Here's how the part is built. I have some questions about the finished solid (model axes, mm). Face numbers are marked on the shaded views. A direction names the side the tool comes from. Coordinates: 2 decimals unless noted, no trailing zeros. Write each loop counter-clockwise with the first axis right and the second up, starting at its lowest first coordinate (ties: lowest second). Pieces come first, ordered by that corner, then holes.
```python
from build123d import *

# Parameters (mm, degrees)
SKETCH1_R           = 2.413
BOSS_EXTRUDE1_DEPTH = 6.35


with BuildPart() as part:
    # Sketch1 → Boss-Extrude1 (new body)
    with BuildSketch(Plane(origin=(0, 0, 0), x_dir=(1, 0, 0), z_dir=(0, 1, 0))):
        Polygon((-44.45, -12.7), (-31.75, -12.7), (-25.4, -12.7), (-25.4, -19.05), (-12.7, -19.05), (-12.7, -12.7), (0, -12.7), (0, -19.05), (12.7, -19.05), (12.7, -12.7), (31.75, -12.7), (31.75, 12.7), (12.7, 12.7), (12.7, 19.05), (0, 19.05), (0, 12.7), (-12.7, 12.7), (-12.7, 19.05), (-25.4, 19.05), (-25.4, 12.7), (-31.75, 12.7), (-44.45, 12.7), align=None)
        with Locations((-6.35, 0)):
            Circle(SKETCH1_R, mode=Mode.SUBTRACT)
    extrude(amount=BOSS_EXTRUDE1_DEPTH)


solid = part.part
```
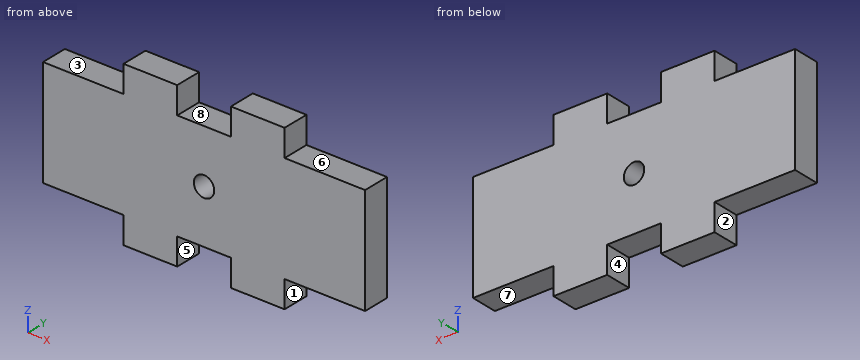
1) On a 3-axis mill with a long thin cutter (end or side, diameter ignored), from which of +Z, -Z, +X, -X, +Y, -Y can I reach the whole of each face in a straight line? I mean the marked faces 5, 6, 7 and 8. Say none if no direction works.
Values follow:
face 5: -Z, +Y, -Y
face 6: +Z, +X, +Y, -Y
face 7: -Z, +X, +Y, -Y
face 8: +Z, +Y, -Y
2) We'd pull the mould along X, two halves only. Please class the marked faces 1, 2, 3 and 4: pulls with the +X half, pulls with the -X half, needs draft (parallel to the pull), parting line crosses it, or undercut.
Values follow:
face 1: pulls with the +X half
face 2: pulls with the -X half
face 3: needs draft
face 4: undercut
3) I need wall thicknesses on probe 1 along X at (y, z) = (2.75, 13); probe 2 along Z at (x, y) = (-6.35, 1.5); probe 3 along X at (y, z) = (2, 0). Which ranges of each line are inside material? Lowest first, please.
Values follow:
probe 1: x = -25.4 to -12.7, 0 to 12.7
probe 2: z = -12.7 to -2.41, 2.41 to 12.7
probe 3: x = -44.45 to -8.76, -3.94 to 31.75
4) Imagine slicing it at B-B on z = 16. Please give me the cut outline in (x, y).
Values follow:
outline: (-25.4, 0) - (-12.7, 0) - (-12.7, 6.35) - (-25.4, 6.35) - close; (0, 0) - (12.7, 0) - (12.7, 6.35) - (0, 6.35) - close
5) Will these pins go through, and if not, where does the flat tip stop? pin 1 (5 mm diameter, centred on x = -32, z = 11.5, fed in from -Y); pin 2 (1.5 mm diameter, centred on x = 13.5, y = 2, fed in from -Z); pin 3 (3 mm diameter, centred on y = 3.5, z = 16.5, fed in from +X); pin 4 (1.9 mm diameter, centred on x = -36, y = 2, fed in from +Z).
Values follow:
pin 1: stops at y = 0
pin 2: stops at z = -12.7
pin 3: stops at x = 12.7
pin 4: stops at z = 12.7
6) Imagine slicing it at A-A on x = -6.35. Please give me the cut outline in (y, z), then the cut area to 3 significant figures.
Values follow:
outline: (0, -12.7) - (6.35, -12.7) - (6.35, -2.41) - (0, -2.41) - close; (0, 2.41) - (6.35, 2.41) - (6.35, 12.7) - (0, 12.7) - close
area: 131 mm2
7) Imagine slicing it at C-C on y = 2.25. Please give me the cut outline in (x, z), then the cut area to 3 significant figures.
Values follow:
outline: (-44.45, -12.7) - (-25.4, -12.7) - (-25.4, -19.05) - (-12.7, -19.05) - (-12.7, -12.7) - (0, -12.7) - (0, -19.05) - (12.7, -19.05) - (12.7, -12.7) - (31.75, -12.7) - (31.75, 12.7) - (12.7, 12.7) - (12.7, 19.05) - (0, 19.05) - (0, 12.7) - (-12.7, 12.7) - (-12.7, 19.05) - (-25.4, 19.05) - (-25.4, 12.7) - (-44.45, 12.7) - close; hole circle Ø4.83 at (-6.35, 0)
area: 2,240 mm2
